Input: part model. Units: mm. Frame: model coordinates. Give positions to 0.01 mm unless a question says otherwise; leave off trailing zeros. Loops run counter-clockwise (first coordinate to the right, second up) from the corner with the lowest first, then second, coordinate; pieces in that order, holes last. Notation, with made-up numbers: (33.25, 75.5) - (85.25, 75.5) arc R28 cw to (85.25, 93.5) - close; hole circle Ø7 at (24.5, 55.25). An arc over 180 degrees is marked (long way). Answer as a JSON object with one key per item and string values.
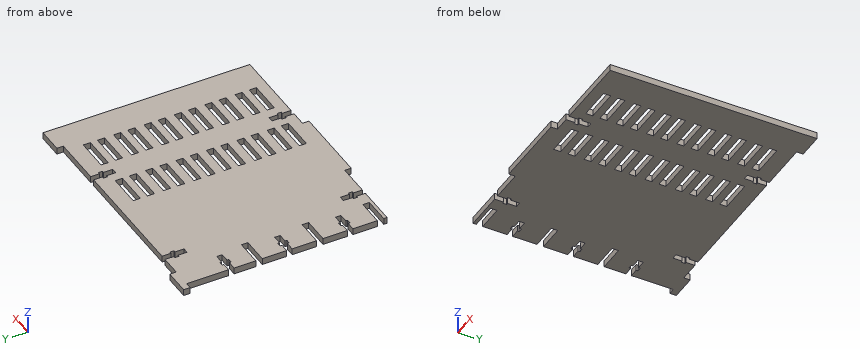
from build123d import *

# Parameters (mm, degrees)
SKETCH1_W           = 25.5
SKETCH1_H           = 5.5
BOSS_EXTRUDE1_DEPTH = 5
CUT_EXTRUDE3_DEPTH  = 10
SKETCH5_W           = 60
SKETCH5_H           = 5
BOSS_EXTRUDE2_DEPTH = 5
SKETCH6_W           = 20.4
SKETCH6_H           = 5
CUT_EXTRUDE4_DEPTH  = 10


with BuildPart() as part:
    # Sketch1 → Boss-Extrude1 (new body)
    with BuildSketch(Plane.XY):
        Polygon((-155.2, 151.5), (-155.2, 146.5), (5.2, 146.5), (5.2, 151.5), (25, 151.5), (25, -8.5), (-170, -8.5), (-170, -6), (-150, -6), (-150, -1), (-170, -1), (-170, 17.9), (-163.2, 17.9), (-163.2, 16.5), (-160, 16.5), (-160, 17.9), (-153, 17.9), (-153, 22.1), (-160, 22.1), (-160, 23.5), (-163.2, 23.5), (-163.2, 22.1), (-170, 22.1), (-170, 41), (-150, 41), (-150, 46), (-170, 46), (-170, 64.9), (-163.2, 64.9), (-163.2, 63.5), (-160, 63.5), (-160, 64.9), (-153, 64.9), (-153, 69.1), (-160, 69.1), (-160, 70.5), (-163.2, 70.5), (-163.2, 69.1), (-170, 69.1), (-170, 88), (-150, 88), (-150, 93), (-170, 93), (-170, 109.8), (-163.2, 109.8), (-163.2, 108.4), (-160, 108.4), (-160, 109.8), (-153, 109.8), (-153, 114), (-160, 114), (-160, 115.4), (-163.2, 115.4), (-163.2, 114), (-170, 114), (-170, 146.5), (-175, 146.5), (-175, 151.5), align=None)
        with Locations((-58.25, 13.75)):
            Rectangle(SKETCH1_W, SKETCH1_H, mode=Mode.SUBTRACT)
        with Locations((-12.75, 2.75)):
            Rectangle(SKETCH1_W, SKETCH1_H, mode=Mode.SUBTRACT)
        with Locations((-58.25, 2.75)):
            Rectangle(SKETCH1_W, SKETCH1_H, mode=Mode.SUBTRACT)
        with Locations((-12.75, 13.75)):
            Rectangle(SKETCH1_W, SKETCH1_H, mode=Mode.SUBTRACT)
        with Locations((-12.75, 26.25)):
            Rectangle(SKETCH1_W, SKETCH1_H, mode=Mode.SUBTRACT)
        with Locations((-58.25, 26.25)):
            Rectangle(SKETCH1_W, SKETCH1_H, mode=Mode.SUBTRACT)
        with Locations((-58.25, 37.25)):
            Rectangle(SKETCH1_W, SKETCH1_H, mode=Mode.SUBTRACT)
        with Locations((-12.75, 37.25)):
            Rectangle(SKETCH1_W, SKETCH1_H, mode=Mode.SUBTRACT)
        with Locations((-12.75, 49.75)):
            Rectangle(SKETCH1_W, SKETCH1_H, mode=Mode.SUBTRACT)
        with Locations((-58.25, 49.75)):
            Rectangle(SKETCH1_W, SKETCH1_H, mode=Mode.SUBTRACT)
        with Locations((-58.25, 60.75)):
            Rectangle(SKETCH1_W, SKETCH1_H, mode=Mode.SUBTRACT)
        with Locations((-12.75, 60.75)):
            Rectangle(SKETCH1_W, SKETCH1_H, mode=Mode.SUBTRACT)
        with Locations((-12.75, 73.25)):
            Rectangle(SKETCH1_W, SKETCH1_H, mode=Mode.SUBTRACT)
        with Locations((-58.25, 73.25)):
            Rectangle(SKETCH1_W, SKETCH1_H, mode=Mode.SUBTRACT)
        with Locations((-58.25, 84.25)):
            Rectangle(SKETCH1_W, SKETCH1_H, mode=Mode.SUBTRACT)
        with Locations((-12.75, 84.25)):
            Rectangle(SKETCH1_W, SKETCH1_H, mode=Mode.SUBTRACT)
        with Locations((-12.75, 96.75)):
            Rectangle(SKETCH1_W, SKETCH1_H, mode=Mode.SUBTRACT)
        with Locations((-58.25, 96.75)):
            Rectangle(SKETCH1_W, SKETCH1_H, mode=Mode.SUBTRACT)
        with Locations((-58.25, 107.75)):
            Rectangle(SKETCH1_W, SKETCH1_H, mode=Mode.SUBTRACT)
        with Locations((-12.75, 107.75)):
            Rectangle(SKETCH1_W, SKETCH1_H, mode=Mode.SUBTRACT)
        with Locations((-12.75, 120.25)):
            Rectangle(SKETCH1_W, SKETCH1_H, mode=Mode.SUBTRACT)
        with Locations((-58.25, 120.25)):
            Rectangle(SKETCH1_W, SKETCH1_H, mode=Mode.SUBTRACT)
        with Locations((-58.25, 131.25)):
            Rectangle(SKETCH1_W, SKETCH1_H, mode=Mode.SUBTRACT)
        with Locations((-12.75, 131.25)):
            Rectangle(SKETCH1_W, SKETCH1_H, mode=Mode.SUBTRACT)
    extrude(amount=BOSS_EXTRUDE1_DEPTH)

    # Sketch4 → Cut-Extrude3 (cut)
    with BuildSketch(Plane.XY.offset(5)):
        Polygon((-33.6, 146.5), (-33.6, 139.7), (-32.2, 139.7), (-32.2, 136.5), (-33.6, 136.5), (-33.6, 129.5), (-37.8, 129.5), (-37.8, 136.5), (-39.2, 136.5), (-39.2, 139.7), (-37.8, 139.7), (-37.8, 146.5), align=None)
        Polygon((-135, 129.5), (-139.2, 129.5), (-139.2, 136.5), (-140.6, 136.5), (-140.6, 139.7), (-139.2, 139.7), (-139.2, 146.5), (-135, 146.5), (-135, 139.7), (-133.6, 139.7), (-133.6, 136.5), (-135, 136.5), align=None)
        Polygon((-33.6, -8.5), (-37.8, -8.5), (-37.8, -1.7), (-39.2, -1.7), (-39.2, 1.5), (-37.8, 1.5), (-37.8, 8.5), (-33.6, 8.5), (-33.6, 1.5), (-32.2, 1.5), (-32.2, -1.7), (-33.6, -1.7), align=None)
        Polygon((-135, -8.5), (-139.2, -8.5), (-139.2, -1.7), (-140.6, -1.7), (-140.6, 1.5), (-139.2, 1.5), (-139.2, 8.5), (-135, 8.5), (-135, 1.5), (-133.6, 1.5), (-133.6, -1.7), (-135, -1.7), align=None)
    extrude(amount=-CUT_EXTRUDE3_DEPTH, mode=Mode.SUBTRACT)

    # Sketch5 → Boss-Extrude2 (add)
    with BuildSketch(Plane.XY.offset(5)):
        with Locations((-80, -11)):
            Rectangle(SKETCH5_W, SKETCH5_H)
    extrude(amount=-BOSS_EXTRUDE2_DEPTH)

    # Sketch6 → Cut-Extrude4 (cut)
    with BuildSketch(Plane.XY.offset(5)):
        with Locations((-159.8, -3.5)):
            Rectangle(SKETCH6_W, SKETCH6_H)
        with Locations((-159.8, 43.5)):
            Rectangle(SKETCH6_W, SKETCH6_H)
        with Locations((-159.8, 90.5)):
            Rectangle(SKETCH6_W, SKETCH6_H)
    extrude(amount=-CUT_EXTRUDE4_DEPTH, mode=Mode.SUBTRACT)


solid = part.part
Item 1: Cut plane D-D (x = 9.5). Return loops of the section in (y, z), then the cut area to 3 significant figures.
Geometry check:
{"outline": "(-8.5, 0) - (151.5, 0) - (151.5, 5) - (-8.5, 5) - close", "area": "800 mm2"}
Item 2: Contact query for flat-ended pins moving along their axis: P1, Ø2.5, axis at x = -56, z = 1.5, coming from the +Y side; P2, Ø1, axis at x = -161.5, z = 2, coming from the -Y side; P3, Ø1, axis at x = -51, y = 72, coming from the +Z side; P4, Ø2.5, axis at y = 84, z = 2, coming from the -X side. Output: stop coordinate, or through.
Geometry check:
{"P1": "stops at y = 146.5", "P2": "stops at y = -8.5", "P3": "passes through", "P4": "stops at x = -170"}
Item 3: Cut plane A-A (y = 84). Return loops of the section in (x, z), then the cut area to 3 significant figures.
Geometry check:
{"outline": "(-170, 0) - (-71, 0) - (-71, 5) - (-170, 5) - close; (-45.5, 0) - (-25.5, 0) - (-25.5, 5) - (-45.5, 5) - close; (0, 0) - (25, 0) - (25, 5) - (0, 5) - close", "area": "720 mm2"}
Item 4: Cut plane B-B (x = -56.5). Give the number of separate pieces and of enclosed holes in the cut face, then the cut area to 3 significant figures.
Geometry check:
{"separate pieces": "13", "enclosed holes": "0", "area": "470 mm2"}
Item 5: Material intervals for line 1 (X direction, y = 4.5, z = 1.25); line 2 (X direction, y = 96.5, z = 4.2); line 3 (X direction, y = 6.5, z = 3.35), sorted ascending. Write a range as [from, to].
Geometry check:
{"line 1": "x = [-170, -139.2], [-135, -71], [-45.5, -37.8], [-33.6, -25.5], [0, 25]", "line 2": "x = [-170, -71], [-45.5, -25.5], [0, 25]", "line 3": "x = [-170, -139.2], [-135, -37.8], [-33.6, 25]"}
